Verification items for the finished model (mm, model axes). A direction names the side the tool comes from. Give positions to 0.01 mm unless a question says otherwise; leave off trailing zeros. Order: outer loops, then holes, each group sorted by start corner. A loop starts at its lowest first (then second) coordinate and runs counter-clockwise, first axis right, second up. Notation, with made-up numbers: (71.25, 30.5) - (85.25, 30.5) arc R10 cw to (85.25, 34.5) - close; hole circle Ø4 at (30, 19.25). An arc over 180 degrees is marked (long way). Answer as a JSON object with one key per item and string values.
```python
from build123d import *

# Parameters (mm, degrees)
F0_R     = 254
F0_R_2   = 244.5
F1_DEPTH = 600
F3_DEPTH = 450


with BuildPart() as f1:
    # F0 (on Front) → F1 (new body, symmetric)
    with BuildSketch(Plane.XZ):
        Circle(F0_R)
        Circle(F0_R_2, mode=Mode.SUBTRACT)
    extrude(amount=F1_DEPTH, both=True)

    # F2 (on Front) → F3 (cut, symmetric)
    with BuildSketch(Plane.XZ):
        with BuildLine():
            ThreePointArc((237.1294283303, -91.0254591845), (209.32805191, 143.8671841789), (0, 254))
            Line((0, 254), (0, 244.5))
            ThreePointArc((0, 244.5), (201.4988531181, 138.4863249281), (228.2604142786, -87.6209636638))
            Line((228.2604142786, -87.6209636638), (237.1294283303, -91.0254591845))
        make_face()
        with BuildLine():
            ThreePointArc((228.2604142786, -87.6209636638), (201.4988531181, 138.4863249281), (0, 244.5))
            Line((0, 244.5), (0, 0))
            Line((0, 0), (228.2604142786, -87.6209636638))
        make_face()
    extrude(amount=F3_DEPTH, both=True, mode=Mode.SUBTRACT)


solid = f1.part
```
(1) Material ranges on line 1 along Y through (x, z) = (233, 91.5); line 2 along X through (y, z) = (-209, 1.5); line 3 along X through (y, z) = (505.5, 158), recorded low to high. Write a range as [from, to].
Computed values:
{"line 1": "y = [-600, -450], [450, 600]", "line 2": "x = [-254, -244.5]", "line 3": "x = [-198.88, -186.59], [186.59, 198.88]"}
(2) Access from +Z, -Z, +X, -X, +Y, -Y to the whole of each face (thin tool, end or side, straight path). Record for faces 1 (the flat face through (-133, 600, 208)), 2 (the flat face through (202, -450, 146)).
Computed values:
{"face 1": "+Z, -Z, +X, -X, +Y", "face 2": "+Z, +X"}
(3) Section check A-A (z = 0). Record the cut outline in (x, y).
Computed values:
{"outline": "(-254, -600) - (-244.5, -600) - (-244.5, 600) - (-254, 600) - close; (244.5, -600) - (254, -600) - (254, -450) - (244.5, -450) - close; (244.5, 450) - (254, 450) - (254, 600) - (244.5, 600) - close"}
(4) Section check D-D (y = -405). Record the cut outline in (x, z), then the cut area to 3 significant figures.
Computed values:
{"outline": "(0, 244.5) - (0, 254) arc R254 ccw (long way) to (237.13, -91.03) - (228.26, -87.62) arc R244.5 cw (long way) to start", "area": "10,300 mm²"}
(5) Gauge pin test, flat ends, axial feed: pin 1 Ø10 at (y, z) = (-322.5, 144) entering from -X; pin 2 Ø1 at (x, y) = (186.5, 81.5) entering from +Z; pin 3 Ø3 at (y, z) = (81, 247) entering from +X. Record the tip position at first contact, or that the pin passes through.
Computed values:
{"pin 1": "stops at x = -212.59", "pin 2": "stops at z = -157.52", "pin 3": "stops at x = 0"}
(6) Release check for a two-part mould opening along Z. For faces 3 (the cylindrical face through (-201.566, -8.4, -154.555)), 4 (the cylindrical face through (-194.03, 8.4, -148.77)), 5 (the flat face through (202, 450, 146)) record: pulls with the +Z half, pulls with the -Z half, needs draft (parallel to the pull), parting line crosses it, or undercut.
Computed values:
{"face 3": "parting line crosses it", "face 4": "undercut", "face 5": "needs draft"}
(7) Section check C-C (x = 167). Record the cut outline in (y, z).
Computed values:
{"outline": "(-600, -191.38) - (600, -191.38) - (600, -178.58) - (-600, -178.58) - close; (-600, 178.58) - (-450, 178.58) - (-450, 191.38) - (-600, 191.38) - close; (450, 178.58) - (600, 178.58) - (600, 191.38) - (450, 191.38) - close"}
(8) Section check B-B (x = -186.5). Record the cut outline in (y, z), then the cut area to 3 significant figures.
Computed values:
{"outline": "(-600, -172.43) - (600, -172.43) - (600, -158.11) - (-600, -158.11) - close; (-600, 158.11) - (600, 158.11) - (600, 172.43) - (-600, 172.43) - close", "area": "34,400 mm²"}
